Model file for the job. Use its own axes, mm. Face numbers are marked on the shaded views. A direction names the side the tool comes from. Give positions to 0.01 mm unless a question says otherwise; leave off trailing zeros. Write each loop counter-clockwise with the first axis right and the second up, starting at its lowest first coordinate (ties: lowest second). Pieces come first, ordered by that corner, then holes. Notation, with made-up numbers: (15, 82) - (64, 82) arc R25 ccw to (64, 94) - close; hole circle Ø9 at (-37.5, -11.5). An arc over 180 degrees is marked (long way). One line per item, written item: value. Start each with the question number.
(1) Mould opens along X. For the marked faces 1, 2 and 3 say: pulls with the +X half, pulls with the -X half, needs draft (parallel to the pull), parting line crosses it, or undercut.
(2) Probe L1, parallel to X at y = 0, z = 3; L2, parallel to Z at x = 3.25, y = -1.5; L3, parallel to X at y = -1, z = 2.75. List the from-to ranges inside material, lowest first.
(3) Cut at A-A, the plane x = 21.25. List the corners of the cut face in (y, z), and give its area (3 significant figures).
(4) Drop flat-ended pins along their axis: P1, Ø8.5, axis at x = 19, y = 2, coming from the +Z side; P2, Ø4, axis at x = 20.5, z = -3, coming from the -Y side; P3, Ø4.5, axis at x = 19.84, y = 0, coming from the +Z side; P4, Ø5, axis at x = 10.5, z = -4, coming from the -Y side. Give the stop position or say it passes through.
(5) 3-axis set-ups, long thin cutter, end or side, ignore diameter. For the marked faces 4, 5 and 6: which of +Z, -Z, +X, -X, +Y, -Y reach the whole face in a straight line?
(6) Cut at B-B, the plane x = 5. List the corners of the cut face in (y, z).
(7) Cut at C-C, the plane x = 16.5. List the corners of the cut face in (y, z), and give its area (3 significant figures).
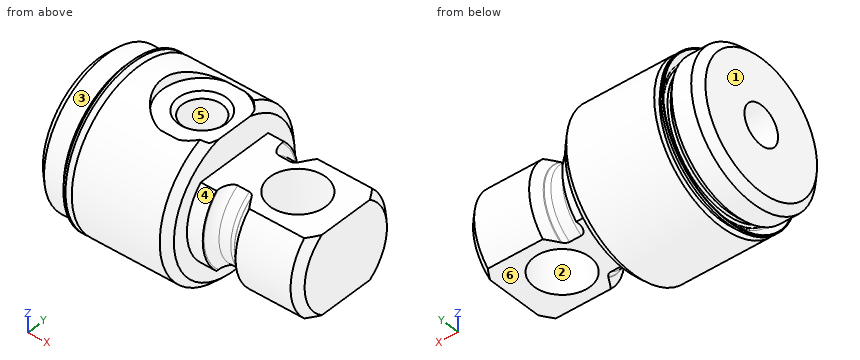
Autodesk Inventor part; units mm, degrees
ref_plane "1_XY" through (15.0876, 0, 0) normal (1, 0, 0) x (0, 0, -1)
ref_plane "1_YZ" through (15.0876, 0, 0) normal (0, 0, -1) x (0, 1, 0)
ref_plane "1_ZX" through (15.0876, 0, 0) normal (0, 1, 0) x (1, 0, 0)
sketch "Sketch_18" plane through (0, 0, 0) normal (0, 0, 1) x (1, 0, 0)
  line L0 (13.5128, 0) -> (0, 0)
  line L1 (0, 0) -> (0, 6.5088)
  line L2 (0, 6.5088) -> (0.762, 7.2708)
  line L3 (0.762, 7.2708) -> (2.7178, 7.2708)
  line L4 (2.7178, 7.2708) -> (3.3528, 6.6357)
  line L5 (3.3528, 6.6357) -> (3.9878, 6.6357)
  line L6 (3.9878, 6.6357) -> (3.9878, 7.8105)
  line L7 (3.9878, 7.8105) -> (12.7508, 7.8105)
  line L8 (12.7508, 7.8105) -> (13.5128, 7.0485)
  line L9 (13.5128, 7.0485) -> (13.5128, 0)
  line L10 (13.5128, 0) -> (0, 0)
revolve "Revolution1" add sketch "Sketch_18" angle 360 about axis through (13.5128, 0, 0) along (1, 0, 0)
sketch "Sketch_15" plane through (0, 0, 0) normal (0, 0, 1) x (1, 0, 0)
  line L0 (24.6126, 0) -> (13.5128, 0)
  line L1 (13.5128, 0) -> (13.5128, 5.5309)
  line L2 (13.5128, 5.5309) -> (15.0876, 5.5309)
  line L3 (15.0876, 5.5309) -> (15.0876, 5.3721)
  arc A0 (15.0876, 5.3721) -> (15.8877, 4.572) centre (15.8877, 5.3721) ccw
  line L4 (15.8877, 4.572) -> (17.0561, 4.572)
  arc A1 (17.0561, 4.572) -> (17.559, 4.7498) centre (17.0561, 5.3721) ccw
  line L5 (17.559, 4.7498) -> (17.6219, 4.8006)
  line L6 (17.6219, 4.8006) -> (18.3775, 5.5563)
  line L7 (18.3775, 5.5563) -> (23.857, 5.5563)
  line L8 (23.857, 5.5563) -> (24.6126, 4.8006)
  line L9 (24.6126, 4.8006) -> (24.6126, 0)
  line L10 (24.6126, 0) -> (13.5128, 0)
revolve "Revolution2" add sketch "Sketch_15" angle 360 about axis through (24.6126, 0, 0) along (1, 0, 0)
sketch "Sketch_9" plane through (24.6126, 0, 0) normal (1, 0, 0) x (0, 0, -1)
  line L0 (-15.621, -31.242) -> (15.621, -31.242)
  line L1 (15.621, -31.242) -> (15.621, 31.242)
  line L2 (15.621, 31.242) -> (-15.621, 31.242)
  line L3 (-15.621, 31.242) -> (-15.621, -31.242)
  line L4 (-3.8989, -15.621) -> (3.8989, -15.621)
  line L5 (3.8989, -15.621) -> (3.8989, 15.621)
  line L6 (3.8989, 15.621) -> (-3.8989, 15.621)
  line L7 (-3.8989, 15.621) -> (-3.8989, -15.621)
extrude "Extrusion1" cut sketch "Sketch_9" against normal blind 11.0998
sketch "Sketch4" plane through (0, 0, 0) normal (-1, 0, 0) x (0, 0, 1)
  point P0 (0, 0)
hole "Hole1" at (0, 0, 0) direction (1, 0, 0) diameter 3.9116 depth 12.2936 tip angle 120
sketch "Sketch_16" plane through (0, 0, 0) normal (0, 1, 0) x (-1, 0, 0)
  line L0 (-10.3124, 7.8105) -> (-10.3124, 0)
  line L1 (-10.3124, 0) -> (-12.2961, 0)
  line L2 (-12.2961, 0) -> (-12.2961, 6.3652)
  line L3 (-12.2961, 6.3652) -> (-12.7254, 6.7945)
  line L4 (-12.7254, 6.7945) -> (-14.2748, 6.7945)
  line L5 (-14.2748, 6.7945) -> (-14.2748, 7.8105)
  line L6 (-14.2748, 7.8105) -> (-10.3124, 7.8105)
  line L7 (-10.3124, 7.8105) -> (-10.3124, 0)
revolve "Revolution3" cut sketch "Sketch_16" angle 360 about axis through (10.3124, 0, 7.8105) along (0, 0, 1)
thread "Thread1"
sketch "Sketch_24" plane through (0, 0, 0) normal (0, 0, 1) x (1, 0, 0)
  line L0 (3.9878, 0) -> (3.3528, 0)
  line L1 (3.1602, 7.8105) -> (3.1602, 7.7263)
  line L2 (3.1602, 7.7263) -> (3.8708, 7.0158)
  arc A0 (3.8708, 6.8362) -> (3.8708, 7.0158) centre (3.781, 6.926) ccw
  line L3 (3.8708, 6.8362) -> (3.6703, 6.6357)
  line L4 (3.6703, 6.6357) -> (3.3528, 6.6357)
  line L5 (3.3528, 6.6357) -> (3.3528, 6.3818)
  line L6 (3.3528, 6.3818) -> (3.9878, 6.3818)
  line L7 (3.9878, 6.3818) -> (3.9878, 7.1861)
  line L8 (3.9878, 7.1861) -> (3.3634, 7.8105)
  line L9 (3.3634, 7.8105) -> (3.1602, 7.8105)
revolve "Revolution4" add sketch "Sketch_24" angle 360 about axis through (3.9878, 0, 0) along (1, 0, 0)
sketch "Sketch_43" plane through (0, 0, 0) normal (0, 0, 1) x (1, 0, 0)
  circle A0 centre (19.8374, 0) radius 2.775
extrude "Extrusion2" cut sketch "Sketch_43" along normal mid plane 11.6967
ref_plane "1_XY" through (15.0876, 0, 0) normal (1, 0, 0) x (0, 0, -1)
ref_plane "1_YZ" through (15.0876, 0, 0) normal (0, 0, -1) x (0, 1, 0)
ref_plane "1_ZX" through (15.0876, 0, 0) normal (0, 1, 0) x (1, 0, 0)
ref_plane "c1_XY" through (13.5128, 5.5309, 0) normal (0, 0, 1) x (1, 0, 0)
ref_plane "c1_YZ" through (13.5128, 5.5309, 0) normal (1, 0, 0) x (0, 1, 0)
ref_plane "c1_ZX" through (13.5128, 5.5309, 0) normal (0, 1, 0) x (0, 0, 1)
ref_plane "c2_XY" through (13.5128, -5.5309, 0) normal (0, 0, 1) x (1, 0, 0)
ref_plane "c2_YZ" through (13.5128, -5.5309, 0) normal (1, 0, 0) x (0, 1, 0)
ref_plane "c2_ZX" through (13.5128, -5.5309, 0) normal (0, 1, 0) x (0, 0, 1)
ref_plane "cc1_XY" through (13.5128, 0, 0) normal (0, 0, 1) x (1, 0, 0)
ref_plane "cc1_YZ" through (13.5128, 0, 0) normal (1, 0, 0) x (0, 1, 0)
ref_plane "cc1_ZX" through (13.5128, 0, 0) normal (0, 1, 0) x (0, 0, 1)
ref_plane "cc2_XY" through (15.0876, 0, 0) normal (0, 0, 1) x (1, 0, 0)
ref_plane "cc2_YZ" through (15.0876, 0, 0) normal (1, 0, 0) x (0, 1, 0)
ref_plane "cc2_ZX" through (15.0876, 0, 0) normal (0, 1, 0) x (0, 0, 1)
ref_plane "lovra1_XY" through (19.9644, 0, 0) normal (1, 0, 0) x (0, 0, -1)
ref_plane "lovra1_YZ" through (19.9644, 0, 0) normal (0, 0, -1) x (0, 1, 0)
ref_plane "lovra1_ZX" through (19.9644, 0, 0) normal (0, 1, 0) x (1, 0, 0)
ref_plane "lovra2_XY" through (19.9644, 6.2865, 0) normal (1, 0, 0) x (0, 0, -1)
ref_plane "lovra2_YZ" through (19.9644, 6.2865, 0) normal (0, 0, -1) x (0, 1, 0)
ref_plane "lovra2_ZX" through (19.9644, 6.2865, 0) normal (0, 1, 0) x (1, 0, 0)
ref_plane "lovra21_XY" through (0, 0, 5.2705) normal (1, 0, 0) x (0, 0, -1)
ref_plane "lovra21_YZ" through (0, 0, 5.2705) normal (0, 0, -1) x (0, 1, 0)
ref_plane "lovra21_ZX" through (0, 0, 5.2705) normal (0, 1, 0) x (1, 0, 0)
ref_plane "lovra22_XY" through (0, 0, -5.2705) normal (1, 0, 0) x (0, 0, -1)
ref_plane "lovra22_YZ" through (0, 0, -5.2705) normal (0, 0, -1) x (0, 1, 0)
ref_plane "lovra22_ZX" through (0, 0, -5.2705) normal (0, 1, 0) x (1, 0, 0)
ref_plane "lovra3_XY" through (19.9644, -6.2865, 0) normal (1, 0, 0) x (0, 0, -1)
ref_plane "lovra3_YZ" through (19.9644, -6.2865, 0) normal (0, 0, -1) x (0, 1, 0)
ref_plane "lovra3_ZX" through (19.9644, -6.2865, 0) normal (0, 1, 0) x (1, 0, 0)
ref_plane "olen_XY" through (19.8374, 0, 0) normal (1, 0, 0) x (0, 0, -1)
ref_plane "olen_YZ" through (19.8374, 0, 0) normal (0, 0, -1) x (0, 1, 0)
ref_plane "olen_ZX" through (19.8374, 0, 0) normal (0, 1, 0) x (1, 0, 0)
ref_plane "p1_XY" through (24.6126, 0, 3.9624) normal (1, 0, 0) x (0, 0, -1)
ref_plane "p1_YZ" through (24.6126, 0, 3.9624) normal (0, 0, -1) x (0, 1, 0)
ref_plane "p1_ZX" through (24.6126, 0, 3.9624) normal (0, 1, 0) x (1, 0, 0)
ref_plane "p2_XY" through (24.6126, 0, -3.9624) normal (1, 0, 0) x (0, 0, -1)
ref_plane "p2_YZ" through (24.6126, 0, -3.9624) normal (0, 0, -1) x (0, 1, 0)
ref_plane "p2_ZX" through (24.6126, 0, -3.9624) normal (0, 1, 0) x (1, 0, 0)
ref_plane "port_XY" through (10.3124, 0, 0) normal (0, 0, 1) x (1, 0, 0)
ref_plane "port_YZ" through (10.3124, 0, 0) normal (1, 0, 0) x (0, 1, 0)
ref_plane "port_ZX" through (10.3124, 0, 0) normal (0, 1, 0) x (0, 0, 1)
ref_plane "port2_XY" through (24.6126, 0, 0) normal (1, 0, 0) x (0, 0, -1)
ref_plane "port2_YZ" through (24.6126, 0, 0) normal (0, 0, -1) x (0, 1, 0)
ref_plane "port2_ZX" through (24.6126, 0, 0) normal (0, 1, 0) x (1, 0, 0)
ref_plane "thd1_XY" through (24.6126, 0, 5.5563) normal (1, 0, 0) x (0, 0, -1)
ref_plane "thd1_YZ" through (24.6126, 0, 5.5563) normal (0, 0, -1) x (0, 1, 0)
ref_plane "thd1_ZX" through (24.6126, 0, 5.5563) normal (0, 1, 0) x (1, 0, 0)
ref_plane "thd2_XY" through (24.6126, 0, -5.5563) normal (1, 0, 0) x (0, 0, -1)
ref_plane "thd2_YZ" through (24.6126, 0, -5.5563) normal (0, 0, -1) x (0, 1, 0)
ref_plane "thd2_ZX" through (24.6126, 0, -5.5563) normal (0, 1, 0) x (1, 0, 0)
ref_plane "to_mounting_bracket_XY" through (13.5128, 0, 0) normal (1, 0, 0) x (0, 0, -1)
ref_plane "to_mounting_bracket_YZ" through (13.5128, 0, 0) normal (0, 0, -1) x (0, 1, 0)
ref_plane "to_mounting_bracket_ZX" through (13.5128, 0, 0) normal (0, 1, 0) x (1, 0, 0)
ref_plane "to_nut_XY" through (15.0876, 0, 0) normal (1, 0, 0) x (0, 0, -1)
ref_plane "to_nut_YZ" through (15.0876, 0, 0) normal (0, 0, -1) x (0, 1, 0)
ref_plane "to_nut_ZX" through (15.0876, 0, 0) normal (0, 1, 0) x (1, 0, 0)
ref_plane "to_pin_XY" through (19.8374, 0, 0) normal (0, 0, 1) x (1, 0, 0)
ref_plane "to_pin_YZ" through (19.8374, 0, 0) normal (1, 0, 0) x (0, 1, 0)
ref_plane "to_pin_ZX" through (19.8374, 0, 0) normal (0, 1, 0) x (0, 0, 1)
ref_plane "to_screw_XY" through (10.3124, 0, 0) normal (0, 1, 0) x (1, 0, 0)
ref_plane "to_screw_YZ" through (10.3124, 0, 0) normal (1, 0, 0) x (0, 0, -1)
ref_plane "to_screw_ZX" through (10.3124, 0, 0) normal (0, 0, -1) x (0, 1, 0)
ref_plane "to_tube_XY" through (3.3528, 0, 0) normal (1, 0, 0) x (0, 0, -1)
ref_plane "to_tube_YZ" through (3.3528, 0, 0) normal (0, 0, -1) x (0, 1, 0)
ref_plane "to_tube_ZX" through (3.3528, 0, 0) normal (0, 1, 0) x (1, 0, 0)
properties part number "02P0Y000_rear_head"
Answers follow:
1. face 1: pulls with the -X half
1. face 2: undercut
1. face 3: needs draft
2. L1: x = 0 to 8.33, 12.3 to 17.06, 22.61 to 24.61
2. L2: z = -7.67 to -7.49, -6.57 to -1.26, 1.26 to 6.57, 7.49 to 7.67
2. L3: x = 0 to 8.6, 12.03 to 17.25, 22.43 to 24.61
3. outline: (-3.96, -3.9) - (-2.39, -3.9) - (-2.39, 3.9) - (-3.96, 3.9) arc R5.56 ccw to start; (2.39, -3.9) - (3.96, -3.9) arc R5.56 ccw to (3.96, 3.9) - (2.39, 3.9) - close
3. area: 41.6 mm²
4. P1: stops at z = 3.9
4. P2: stops at y = -5.47
4. P3: passes through
4. P4: stops at y = -7.67
5. face 4: -Y
5. face 5: +Z
5. face 6: -Z, +X, +Y, -Y
6. outline: circle Ø15.62 at (0, 0); hole circle Ø3.91 at (0, 0)
7. outline: (-2.39, -3.9) - (2.39, -3.9) arc R4.57 ccw to (2.39, 3.9) - (-2.39, 3.9) arc R4.57 ccw to start
7. area: 61.3 mm²
